Read the model definition and answer for the solid it produces. Units are mm, in the model's axes. Face numbers are marked on the shaded views. A direction names the side the tool comes from. Coordinates: 2 decimals unless noted, no trailing zeros. Write each loop counter-clockwise with the first axis right and the second up, starting at its lowest first coordinate (ties: lowest second). Pieces come first, ordered by that corner, then holes.
(1) The part is cut by section C-C, the plane x = -10.15. Determine the outline of the cut face in (y, z).
(2) Straight lines are drawn through the part: line 1 along Z through (x, y) = (-10.15, 1.1); line 2 along Y through (x, z) = (-20.95, -4); line 3 along Z through (x, y) = (-21.6, 19). For each, find the intervals that lie inside material, in ascending order.
(3) The part is cut by section A-A, the plane y = 9.75. Determine the outline of the cut face in (x, z).
(4) Which of the six approach directions +Z, -Z, +X, -X, +Y, -Y give full straight-line access (tool end or side, diameter ignored) to the marked faces 1 and 2?
(5) Given pin 1 (10 mm diameter, centred on x = -10.15, z = -35.3, fed in from -Y); pin 2 (3.5 mm diameter, centred on y = 1, z = -23.5, fed in from -X); pin 3 (8 mm diameter, centred on x = -17.5, z = -20.5, fed in from +Y); pin 4 (4 mm diameter, centred on y = 10, z = -37.5, fed in from +X), each flat-ended and moving along its own axis, determine where each tip first touches the part or whether it passes through.
(6) The part is cut by section D-D, the plane y = 19. Determine the outline of the cut face in (x, z), and give its area (3 significant figures).
(7) The part is cut by section B-B, the plane z = -24. Determine the outline of the cut face in (x, y), and give its area (3 significant figures).
Autodesk Inventor part; units mm, degrees
ref_plane "YZ Plane" through (0, 0, 0) normal (1, 0, 0) x (0, 1, 0)
ref_plane "XZ Plane" through (0, 0, 0) normal (0, 1, 0) x (-1, 0, 0)
ref_plane "XY Plane" through (0, 0, 0) normal (0, 0, 1) x (1, 0, 0)
sketch "Sketch1" plane through (0, 0, 0) normal (0, 1, 0) x (-1, 0, 0)
  line L0 (0, 0) -> (20.3, 0)
  line L1 (20.3, 0) -> (20.3, -45.3)
  line L2 (20.3, -45.3) -> (0, -45.3)
  line L3 (0, -45.3) -> (0, 0)
  dimension "d0" = 20.3
  dimension "d1" = 45.3
extrude "Extrusion1" add sketch "Sketch1" along normal blind 3
sketch "Sketch2" plane through (0, 3, 0) normal (0, 1, 0) x (1, 0, 0)
  circle A0 centre (-10.15, 10) radius 8.5
  line L0 (-20.3, 45.3) -> (-20.3, 0)
  line L1 (0, 0) -> (0, 45.3)
  line L2 (-20.3, 0) -> (0, 0)
  circle A1 centre (-10.15, 35.3) radius 8.5
  line L3 (0, 45.3) -> (-20.3, 45.3)
  dimension "d4" = 17
  dimension "d5" = 10.15
  dimension "d6" = 10.15
  dimension "d7" = 10
  dimension "d8" = 17
  dimension "d9" = 10.15
  dimension "d10" = 10
extrude "Extrusion2" cut sketch "Sketch2" against normal blind 3 contours A0 | A1
sketch "Sketch3" plane through (-20.3, 0, -45.3) normal (-1, 0, 0) x (0, 0, 1)
  line L0 (45.3, 3) -> (0, 3)
  line L1 (45.3, 0) -> (27.8, 0)
  line L2 (27.8, 0) -> (27.8, 3)
  line L3 (27.8, 3) -> (45.3, 3)
  line L4 (45.3, 3) -> (45.3, 0)
  line L5 (0, 0) -> (17.5, 0)
  line L6 (17.5, 0) -> (17.5, 3)
  line L7 (17.5, 3) -> (0, 3)
  line L8 (0, 3) -> (0, 0)
  point P0 (0, 3)
  dimension "d13" = 17.5
  dimension "d14" = 17.5
extrude "Extrusion3" add sketch "Sketch3" along normal blind 3
sketch "Sketch4" plane through (0, 3, 0) normal (0, 1, 0) x (1, 0, 0)
  line L0 (0, 0) -> (-23.3, 0)
  line L1 (0, 45.3) -> (-23.3, 45.3)
  line L2 (-23.3, 0) -> (-20.3, 0)
  line L3 (-20.3, 0) -> (-20.3, 45.3)
  line L4 (-20.3, 45.3) -> (-23.3, 45.3)
  line L5 (-23.3, 45.3) -> (-23.3, 0)
  dimension "d17" = 3
extrude "Extrusion4" add sketch "Sketch4" along normal blind 20
sketch "Sketch5" plane through (-23.3, 0, -45.3) normal (-1, 0, 0) x (0, 0, 1)
  line L0 (27.8, 0) -> (27.8, 3)
  line L1 (27.8, 3) -> (17.5, 3)
  line L2 (17.5, 3) -> (17.5, 23)
  line L3 (17.5, 23) -> (27.8, 23)
  line L4 (27.8, 23) -> (27.8, 3)
  line L5 (17.5, 0) -> (17.5, 3)
  point P0 (45.3, 0)
  dimension "d20" = 10.3
  dimension "d21" = 0
  dimension "d22" = 20
extrude "Extrusion5" cut sketch "Sketch5" against normal blind 3
sketch "Sketch6" plane through (0, 0, 0) normal (0, -1, 0) x (1, 0, 0)
  line L0 (-3, -28.15) -> (-3, -17.15) construction
  line L1 (-0.5, -25.65) -> (-0.5, -19.65)
  line L2 (-5.5, -19.65) -> (-5.5, -25.65)
  arc A0 (-5.5, -25.65) -> (-0.5, -25.65) centre (-3, -25.65) ccw
  arc A1 (-0.5, -19.65) -> (-5.5, -19.65) centre (-3, -19.65) ccw
  line L3 (0, 0) -> (0, -45.3)
  line L4 (0, -45.3) -> (-23.3, -45.3)
  point P0 (-3, -22.65)
  dimension "d25" = 11
  dimension "d26" = 5
  dimension "d27" = 0.5
  dimension "d28" = 22.65
extrude "Extrusion6" cut sketch "Sketch6" against normal blind 3
sketch "Sketch7" plane through (0, 0, 0) normal (0, -1, 0) x (1, 0, 0)
  line L0 (-20.3, -27.8) -> (-20.3, -17.5)
  line L1 (-20.3, -27.8) -> (-18.3, -27.8)
  line L2 (-18.3, -27.8) -> (-18.3, -17.5)
  line L3 (-18.3, -17.5) -> (-20.3, -17.5)
  line L4 (-20.3, -17.5) -> (-20.3, -27.8)
  point P0 (0, 0)
  dimension "d31" = 2
extrude "Extrusion7" cut sketch "Sketch7" against normal blind 3
sketch "Sketch8" plane through (0, 0, 0) normal (0, -1, 0) x (1, 0, 0)
  line L0 (0, 0) -> (0, -45.3)
  line L1 (0, -45.3) -> (-23.3, -45.3)
  line L2 (0, 0) -> (-23.3, 0)
  point P0 (-2.5, -2.5)
  point P1 (-18.8095, -2.5)
  point P2 (-18.6137, -42.8)
  point P3 (-2.5, -42.8)
  dimension "d52" = 2.5
  dimension "d53" = 2.5
  dimension "d54" = 2.5
  dimension "d55" = 2.5
  dimension "d56" = 2.5
  dimension "d57" = 2.5
hole "Hole1" at (-2.5, 0, -42.8) at (-2.5, 0, -2.5) at (-18.8095, 0, -2.5) at (-18.6137, 0, -42.8) direction (0, 1, 0) diameter 3 depth 3 tip angle 118
sketch "Sketch9" plane through (-23.3, 0, -45.3) normal (-1, 0, 0) x (0, 0, 1)
  line L0 (0, 23) -> (45.3, 23)
  line L1 (0, 0) -> (0, 23)
  line L2 (45.3, 0) -> (45.3, 23)
  point P0 (4, 19)
  point P1 (41.3, 19)
  dimension "d41" = 4
  dimension "d49" = 4
  dimension "d50" = 4
  dimension "d51" = 4
hole "Hole2" at (-23.3, 19, -41.3) at (-23.3, 19, -4) direction (1, 0, 0) diameter 4 depth 3 tip angle 118
properties part number "USSensorBracket"
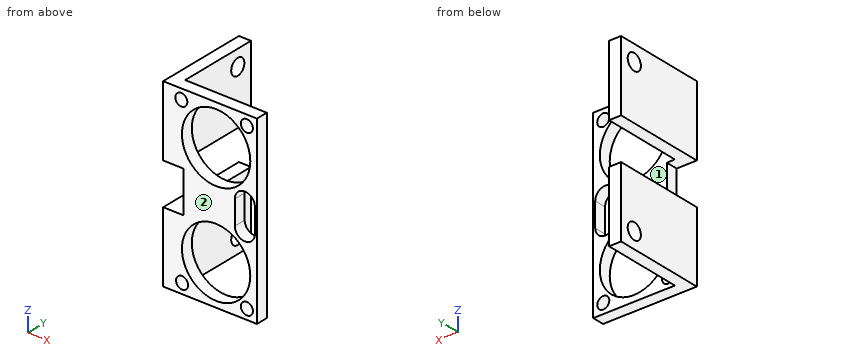
Computed:
1. outline: (0, -45.3) - (3, -45.3) - (3, -43.8) - (0, -43.8) - close; (0, -26.8) - (3, -26.8) - (3, -18.5) - (0, -18.5) - close; (0, -1.5) - (3, -1.5) - (3, 0) - (0, 0) - close
2. line 1: z = -45.3 to -43.8, -26.8 to -18.5, -1.5 to 0
2. line 2: y = 0 to 17, 21 to 23
2. line 3: z = -45.3 to -43.3, -39.3 to -27.8, -17.5 to -6, -2 to 0
3. outline: (-23.3, -45.3) - (-20.3, -45.3) - (-20.3, -27.8) - (-23.3, -27.8) - close; (-23.3, -17.5) - (-20.3, -17.5) - (-20.3, 0) - (-23.3, 0) - close
4. face 1: +Z, -Z, +X, +Y
4. face 2: +Z, -Z, +X, -X, -Y
5. pin 1: passes through
5. pin 2: stops at x = -18.3
5. pin 3: stops at y = 3
5. pin 4: stops at x = -20.3
6. outline: (-23.3, -45.3) - (-20.3, -45.3) - (-20.3, -43.3) - (-23.3, -43.3) - close; (-23.3, -39.3) - (-20.3, -39.3) - (-20.3, -27.8) - (-23.3, -27.8) - close; (-23.3, -17.5) - (-20.3, -17.5) - (-20.3, -6) - (-23.3, -6) - close; (-23.3, -2) - (-20.3, -2) - (-20.3, 0) - (-23.3, 0) - close
6. area: 81.0 mm2
7. outline: (-18.3, 0) - (-5.5, 0) - (-5.5, 3) - (-18.3, 3) - close; (-0.5, 0) - (0, 0) - (0, 3) - (-0.5, 3) - close
7. area: 39.9 mm2
